Drawing for the job (mm, zero at the part's lowest x, y, z). Round coordinates to 2 decimals unless told otherwise and drop trailing zeros. Order: outer loops, then holes, each group sorted by start corner. A loop starts at its lowest first (then second) coordinate and runs counter-clockwise, first axis right, second up. Notation, with made-up numbers: M 59.25,-36.5 L 109.25,-36.5 A37 ccw 109.25,2.5 Z; hole C 39.5,56.5 d5. An arc over 180 degrees is marked long. One line per item, written item: value. Start each with the question number.
Item 1: Band-saw the part on A-A, the plane y = 5. Write the cut outline in (x, z), then the cut area to 3 significant figures.
Item 2: Probe L1, parallel to X at y = 5, z = 1.95; L2, parallel to Y at x = 45, z = 1.1; L3, parallel to X at y = 3.75, z = 0.55. List the from-to ranges inside material, lowest first.
Item 3: Band-saw the part on C-C, the plane z = 1.8. Write the cut outline in (x, y).
Item 4: Band-saw the part on B-B, the plane x = 5. Write the cut outline in (y, z).
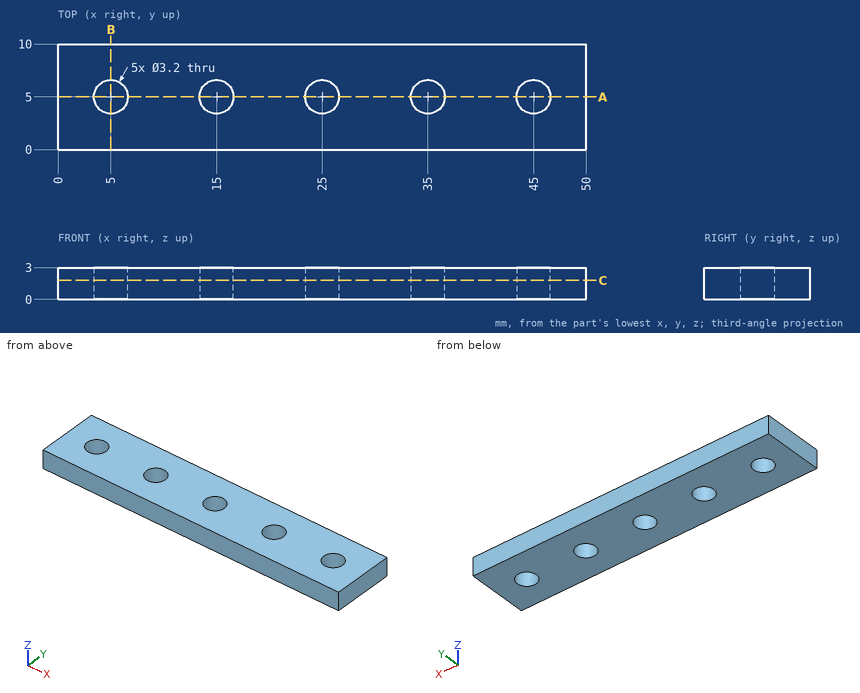
Output:
1. outline: M 0,0 L 3.4,0 L 3.4,3 L 0,3 Z; M 6.6,0 L 13.4,0 L 13.4,3 L 6.6,3 Z; M 16.6,0 L 23.4,0 L 23.4,3 L 16.6,3 Z; M 26.6,0 L 33.4,0 L 33.4,3 L 26.6,3 Z; M 36.6,0 L 43.4,0 L 43.4,3 L 36.6,3 Z; M 46.6,0 L 50,0 L 50,3 L 46.6,3 Z
1. area: 102 mm²
2. L1: x = 0 to 3.4, 6.6 to 13.4, 16.6 to 23.4, 26.6 to 33.4, 36.6 to 43.4, 46.6 to 50
2. L2: y = 0 to 3.4, 6.6 to 10
2. L3: x = 0 to 4, 6 to 14, 16 to 24, 26 to 34, 36 to 44, 46 to 50
3. outline: M 0,0 L 50,0 L 50,10 L 0,10 Z; hole C 5,5 d3.2; hole C 15,5 d3.2; hole C 25,5 d3.2; hole C 35,5 d3.2; hole C 45,5 d3.2
4. outline: M 0,0 L 3.4,0 L 3.4,3 L 0,3 Z; M 6.6,0 L 10,0 L 10,3 L 6.6,3 Z
